Model file for the job. Use its own axes, mm. Face numbers are marked on the shaded views. Round coordinates to 2 decimals unless told otherwise and drop trailing zeros. Loops run counter-clockwise (first coordinate to the right, second up) from the corner with the lowest first, then second, coordinate; pieces in that order, holes last. Notation, with made-up numbers: (30.5, 31.5) -> (71.5, 31.5) arc R28 ccw to (71.5, 67.5) -> close; hole circle Ø8 at (59, -33.75). An arc over 180 degrees is marked (long way). Use a Markdown table: item, result. Add a question column.
```python
from build123d import *

# Parameters (mm, degrees)
ESQUISSE1_R        = 2
BOSS_EXTRU_1_DEPTH = 1
CHANFREIN1_SIZE    = 1


with BuildPart() as part:
    # Esquisse1 → Boss.-Extru.1 (new body)
    with BuildSketch(Plane.XY):
        with BuildLine():
            Line((0, 0), (20, 0))
            ThreePointArc((20, 0), (25, -5), (20, -10))
            Line((20, -10), (0, -10))
            ThreePointArc((0, -10), (-5, -5), (0, 0))
        make_face()
        with Locations((0, -5)):
            Circle(ESQUISSE1_R, mode=Mode.SUBTRACT)
        with Locations((20, -5)):
            Circle(ESQUISSE1_R, mode=Mode.SUBTRACT)
    extrude(amount=BOSS_EXTRU_1_DEPTH)

    # Chanfrein1
    chanfrein1_edges = [part.edges().sort_by_distance(p)[0] for p in [
        (-2, -5, 1),
        (18, -5, 1),
    ]]
    chamfer(chanfrein1_edges, length=CHANFREIN1_SIZE - 0.0001)  # a hair under: the kernel refuses the full size


solid = part.part
```
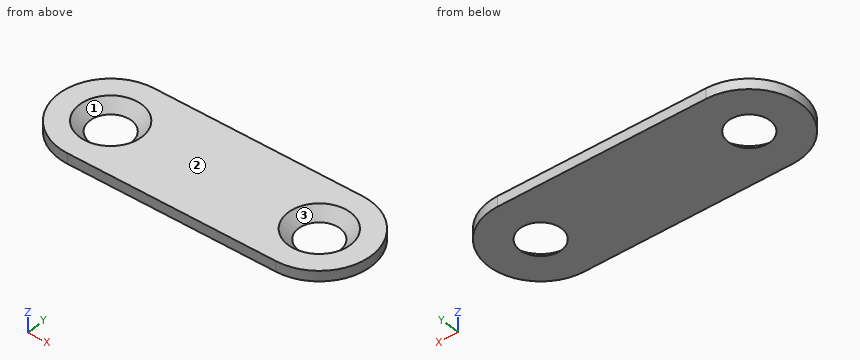
1) Pull direction X, two halves, no side cores. Call the marked faces 1, 2 and 3: +X half, -X half, draft (parallel to the pull), parting line (faces both ways), or undercut.
2) Wall check: probe 1 along X at (y, z) = (-5, 0.05); probe 2 along X at (y, z) = (-7.25, 0.8); probe 3 along Y at (x, z) = (20, 0.05). Give the ranges that are in metal, low to high. Write a range as from..to.
3) Cut at B-B on z = 0.5. Write the cut outline in (x, y).
4) Cut at A-A on y = -5. Count the separate pieces of the cut face and the enclosed holes in it, and give its area (3 significant figures).
Established:
| question | item | result |
|---|---|---|
| 1 | face 1 | undercut |
| 1 | face 2 | draft |
| 1 | face 3 | undercut |
| 2 | probe 1 | x = -5..-2.05, 2.05..17.95, 22.05..25 |
| 2 | probe 2 | x = -4.47..-1.67, 1.67..18.33, 21.67..24.47 |
| 2 | probe 3 | y = -10..-7.05, -2.95..0 |
| 3 | outline | (0, -10) -> (20, -10) arc R5 ccw to (20, 0) -> (0, 0) arc R5 ccw to start; hole circle Ø5 at (0, -5); hole circle Ø5 at (20, -5) |
| 4 | separate pieces | 3 |
| 4 | enclosed holes | 0 |
| 4 | area | 20.0 mm^2 |
